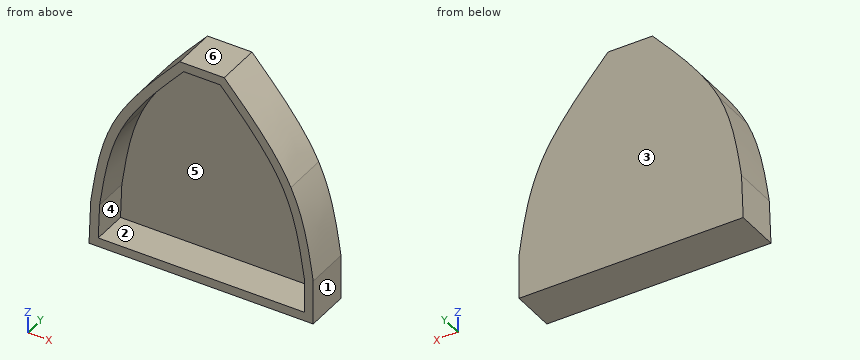
from build123d import *

# Parameters (mm, degrees)
F1_DEPTH = 12.7
F2_T     = -2.54


with BuildPart() as f1:
    # F0 (on Front) → F1 (new body)
    with BuildSketch(Plane.XZ):
        with BuildLine():
            Line((0, 0), (31.75, 0))
            Line((31.75, 0), (31.75, 12.7000007778))
            add(Edge.make_bspline(
                [(25.3999978304, 38.1000004709), (29.2536024334, 30.0036908619), (30.5018012167, 21.3518458199), (31.75, 12.7000007778)],
                knots=[0.5240852488, 0.5240852488, 0.5240852488, 0.5240852488, 1, 1, 1, 1], degree=3))
            Line((25.3999978304, 38.1000004709), (0, 38.1000004709))
            Line((0, 38.1000004709), (0, 0))
        make_face()
        with BuildLine():
            Line((-32.2369039059, 0), (0, 0))
            Line((0, 0), (0, 38.1000004709))
            Line((0, 38.1000004709), (-25.399999693, 38.1000004709))
            add(Edge.make_bspline(
                [(-25.399999693, 38.1000004709), (-29.2536043883, 30.0036909518), (-30.5018027008, 21.3518458648), (-31.7500010133, 12.7000007778)],
                knots=[0.5240852553, 0.5240852553, 0.5240852553, 0.5240852553, 1, 1, 1, 1], degree=3))
            Line((-31.7500010133, 12.7000007778), (-32.2369039059, 0))
        make_face()
        with BuildLine():
            Line((-25.399999693, 38.1000004709), (0, 38.1000004709))
            Line((0, 38.1000004709), (0, 63.5000020266))
            Line((0, 63.5000020266), (-6.3499994576, 63.5000020266))
            add(Edge.make_bspline(
                [(-6.3499994576, 63.5000020266), (-13.7531726904, 55.2578967946), (-21.1563459231, 47.0157915626), (-25.399999693, 38.1000004709)],
                knots=[0, 0, 0, 0, 0.5240852553, 0.5240852553, 0.5240852553, 0.5240852553], degree=3))
        make_face()
        with BuildLine():
            Line((0, 63.5000020266), (0, 38.1000004709))
            Line((0, 38.1000004709), (25.3999978304, 38.1000004709))
            add(Edge.make_bspline(
                [(6.3499999233, 63.5000020266), (13.7531720977, 55.2578967284), (21.1563442721, 47.0157914303), (25.3999978304, 38.1000004709)],
                knots=[0, 0, 0, 0, 0.5240852488, 0.5240852488, 0.5240852488, 0.5240852488], degree=3))
            Line((6.3499999233, 63.5000020266), (0, 63.5000020266))
        make_face()
    extrude(amount=F1_DEPTH)

    # F2
    f2_openings = [f1.faces().sort_by_distance(p)[0] for p in [
        (-0.031333, -12.7, 26.51292),
    ]]
    offset(amount=F2_T, openings=f2_openings, kind=Kind.INTERSECTION)


solid = f1.part
Could you check a few things on this model? Use its own coordinates, in mm. Face numbers are marked on the shaded views. A direction names the side the tool comes from. Coordinates: 2 decimals unless noted, no trailing zeros.
1. For the marked faces 5 and 6, which set-ups out of +Z, -Z, +X, -X, +Y, -Y let a thin tool reach every point of the face, with its end or its side?
2. We'd pull the mould along X, two halves only. Please class the marked faces 1, 2, 3 and 4: released by +X, released by -X, zero draft, split by the parting line, or undercut.
3. I need wall thicknesses on L1, parallel to Z at x = -2, y = -9.25; L2, parallel to Y at x = -14, z = 20.5; L3, parallel to X at y = -5.5, z = 10. Which ranges of each line are inside material? Lowest first, please.
4. For P1, Ø3, axis at y = -9, z = 7, coming from the -X side; P2, Ø10, axis at x = 7, z = 8.5, coming from the -Y side; P3, Ø2, axis at y = -5, z = 28, coming from the +X side, each with a flat end and sliding along its axis, tell me the tip position at first contact or that it passes through.
Computed values:
1. face 5: -Y
1. face 6: +Z, +X, -X, +Y, -Y
2. face 1: released by +X
2. face 2: undercut
2. face 3: zero draft
2. face 4: undercut
3. L1: z = 0 to 2.54, 60.96 to 63.5
3. L2: y = -2.54 to 0
3. L3: x = -31.85 to -29.31, 29.21 to 31.75
4. P1: stops at x = -32.03
4. P2: stops at y = -2.54
4. P3: stops at x = 29.23
